from build123d import *

# Parameters (mm, degrees)
F0_W         = 63.5
F0_H         = 342.9
F0_H_2       = 63.5
F0_W_2       = 241.3
F1_DEPTH     = 165.1
F2_R         = 12.7
F3_R         = 12.7
F4_T1_DEPTH  = 425.45
F4_T3_DEPTH  = 393.7
F4_S7_W      = 12.7
F4_S7_H      = 12.7
F4_T8_DEPTH  = 12.7
F4_S13_W     = 12.7
F4_S13_H     = 12.7
F4_T14_DEPTH = 12.7


# Not quite as in the source:
# - a fillet or chamfer that OpenCascade refuses, or shapes differently, is made with other operations: its cross-section is extruded or revolved along the edge and cut away or added


with BuildPart() as f1:
    # F0 (on Front) → F1 (new body, symmetric)
    with BuildSketch(Plane.XZ):
        with Locations((-120.65, 198.9844056189)):
            Rectangle(F0_W, F0_H)
        with Locations((-120.65, -4.2155943811)):
            Rectangle(F0_W, F0_H_2)
        with Locations((31.75, -4.2155943811)):
            Rectangle(F0_W_2, F0_H_2)
    extrude(amount=F1_DEPTH, both=True)

    # F2
    f2_edges = [f1.edges().sort_by_distance(p)[0] for p in [
        (31.75, -165.1, 27.534406),
        (152.4, 0, 27.534406),
        (31.75, 165.1, 27.534406),
        (-88.9, 0, 27.534406),
        (-88.9, 165.1, 198.984406),
        (-88.9, -165.1, 198.984406),
        (-88.9, 0, 370.434406),
    ]]
    fillet(f2_edges, radius=F2_R)

    # F3
    f3_edges = [f1.edges().sort_by_distance(p)[0] for p in [
        (0, -165.1, -35.965594),
        (152.4, 0, -35.965594),
        (0, 165.1, -35.965594),
        (-152.4, 0, -35.965594),
    ]]
    fillet(f3_edges, radius=F3_R)

    # F4: fillet of radius 12.7 on 3 edges, made by hand

    # F4_s2 → F4_t1 (cut)
    with BuildSketch(Plane.XY.offset(-23.2655943811)):
        with BuildLine():
            ThreePointArc((-152.4, -152.4), (-148.6802561211, -161.3802561211), (-139.7, -165.1))
            Line((-139.7, -165.1), (-152.4, -165.1))
            Line((-152.4, -165.1), (-152.4, -152.4))
        make_face()
        with BuildLine():
            ThreePointArc((-139.7, 165.1), (-148.6802561211, 161.3802561211), (-152.4, 152.4))
            Line((-152.4, 152.4), (-152.4, 165.1))
            Line((-152.4, 165.1), (-139.7, 165.1))
        make_face()
    extrude(amount=F4_T1_DEPTH, mode=Mode.SUBTRACT)

    # F4_s4 → F4_t3 (cut)
    with BuildSketch(Plane.XZ.offset(-196.85)):
        with BuildLine():
            ThreePointArc((-152.4, 357.7344056189), (-148.6802561211, 366.71466174), (-139.7, 370.4344056189))
            Line((-139.7, 370.4344056189), (-152.4, 370.4344056189))
            Line((-152.4, 370.4344056189), (-152.4, 357.7344056189))
        make_face()
    extrude(amount=F4_T3_DEPTH, mode=Mode.SUBTRACT)


with BuildPart() as f4_tool6:
    # F4_s7 → F4_t8 (new body)
    with BuildSketch(Plane.XZ.offset(-152.4)):
        with Locations((-146.05, -29.6155943811)):
            Rectangle(F4_S7_W, F4_S7_H)
    extrude(amount=-F4_T8_DEPTH)

    # F4_s9 → F4_t10 (revolve, cut)
    with BuildSketch(Plane(origin=(-139.7, 152.4, -23.2655943811), x_dir=(0.7071067812, 0, 0.7071067812), z_dir=(-0.7071067812, 0, 0.7071067812))):
        with BuildLine():
            ThreePointArc((0, -12.7), (12.7, 0), (0, 12.7))
            Line((0, 12.7), (0, -12.7))
        make_face()
    revolve(axis=Axis((-139.7, 152.4, -23.2655943811), (0, 1, 0)), mode=Mode.SUBTRACT)


with BuildPart() as f1_1:
    add(f1.part)

    # F4_t5: cut F4_tool6
    add(f4_tool6.part, mode=Mode.SUBTRACT)


with BuildPart() as f4_tool12:
    # F4_s13 → F4_t14 (new body)
    with BuildSketch(Plane.YZ.offset(-139.7)):
        with Locations((-158.75, -29.6155943811)):
            Rectangle(F4_S13_W, F4_S13_H)
    extrude(amount=-F4_T14_DEPTH)

    # F4_s15 → F4_t16 (revolve, cut)
    with BuildSketch(Plane(origin=(-139.7, -152.4, -23.2655943811), x_dir=(0, 0.7071067812, 0.7071067812), z_dir=(0, -0.7071067812, 0.7071067812))):
        with BuildLine():
            ThreePointArc((0, -12.7), (12.7, 0), (0, 12.7))
            Line((0, 12.7), (0, -12.7))
        make_face()
    revolve(axis=Axis((-139.7, -152.4, -23.2655943811), (-1, 0, 0)), mode=Mode.SUBTRACT)


with BuildPart() as f1_2:
    add(f1_1.part)

    # F4_t11: cut F4_tool12
    add(f4_tool12.part, mode=Mode.SUBTRACT)


solid = f1_2.part
Input: part model. Units: mm. Frame: model coordinates. A direction names the side the tool comes from. Coordinates: 2 decimals unless noted, no trailing zeros. Loops run counter-clockwise (first coordinate to the right, second up) from the corner with the lowest first, then second, coordinate; pieces in that order, holes last. Notation, with made-up numbers: (17.25, 27) - (64.25, 27) arc R20 cw to (64.25, 32) - close; hole circle Ø1 at (15.5, 52.5). An arc over 180 degrees is marked (long way). Answer in a Markdown table with one row per item. Add a question column.
Item 1: Access query for faces 4 (the cylindrical face through (-92.52, -161.28, 207.65)), 5 (the flat face through (30, -2, 27.534)), 6 (the cylindrical face through (8.395, -161.478, -32.147)), 7 (the cylindrical face through (-148.778, -2.134, -32.147)), 8 (the cylindrical face through (39.7, 161.281, 23.913)). Directions: +Z, -Z, +X, -X, +Y, -Y. A direction counts if a zero-diameter tool reaches every point of the face in a straight line with its end or side. Return the directions, or none.
Item 2: Mould query, pull axis Z, two halves, no side actions, for faces 1 (the cylindrical face through (8.395, 161.478, -32.147)), 2 (the flat face through (-103, 165.1, 116)), 3 (the flat face through (-121, -2, 370.434)). Classes: released by +Z, released by -Z, zero draft, split by the parting line, or undercut.
Item 3: Contact query for flat-ended pins moving along their axis: P1, Ø6, axis at x = 7.5, y = -8.5, coming from the +Z side; P2, Ø3, axis at y = -125.5, z = 104, coming from the +X side; P3, Ø8, axis at y = -28, z = 16, coming from the +X side. Output: stop coordinate, or through.
Item 4: Line query: line 1 along Z through (x, y) = (73, 97); line 2 along X through (y, z) = (52.5, 278); line 3 along X through (y, z) = (-15, 29). Output: solid intervals per line, ascending. Write a range as [from, to].
Item 5: Section query B-B on z = 153. Return the cut outline in (x, y).
Item 6: Section query A-A on y = -111.5. Return the cut outline in (x, z).
Item 7: Section query C-C on x = 4.5. Return the cut outline in (y, z).
Recorded:
| question | item | result |
|---|---|---|
| 1 | face 4 | +Z, +X, -Y |
| 1 | face 5 | +Z, +X, +Y, -Y |
| 1 | face 6 | -Z, +X, -X, -Y |
| 1 | face 7 | -Z, -X, +Y, -Y |
| 1 | face 8 | +Z, +X, +Y |
| 2 | face 1 | released by -Z |
| 2 | face 2 | zero draft |
| 2 | face 3 | released by +Z |
| 3 | P1 | z = 27.53 |
| 3 | P2 | x = -88.9 |
| 3 | P3 | x = 152.4 |
| 4 | line 1 | [-35.97, 27.53] |
| 4 | line 2 | [-152.4, -88.9] |
| 4 | line 3 | [-152.4, -82.12] |
| 5 | outline | (-152.4, -152.4) arc R12.7 ccw to (-139.7, -165.1) - (-101.6, -165.1) arc R12.7 ccw to (-88.9, -152.4) - (-88.9, 152.4) arc R12.7 ccw to (-101.6, 165.1) - (-139.7, 165.1) arc R12.7 ccw to (-152.4, 152.4) - close |
| 6 | outline | (-152.4, -23.27) arc R12.7 ccw to (-139.7, -35.97) - (139.7, -35.97) arc R12.7 ccw to (152.4, -23.27) - (152.4, 14.83) arc R12.7 ccw to (139.7, 27.53) - (-76.2, 27.53) arc R12.7 cw to (-88.9, 40.23) - (-88.9, 357.73) arc R12.7 ccw to (-101.6, 370.43) - (-139.7, 370.43) arc R12.7 ccw to (-152.4, 357.73) - close |
| 7 | outline | (-165.1, -23.27) arc R12.7 ccw to (-152.4, -35.97) - (152.4, -35.97) arc R12.7 ccw to (165.1, -23.27) - (165.1, 14.83) arc R12.7 ccw to (152.4, 27.53) - (-152.4, 27.53) arc R12.7 ccw to (-165.1, 14.83) - close |
